from build123d import *

# Parameters (mm, degrees)
BOSS_EXTRUDE1_DEPTH = 25.4
SKETCH2_R           = 2.4892
CUT_EXTRUDE1_DEPTH  = 4.175
SKETCH4_R           = 2.4892
CUT_EXTRUDE2_DEPTH  = 16.875


with BuildPart() as part:
    # Sketch1 → Boss-Extrude1 (new body)
    with BuildSketch(Plane.XY):
        Polygon((0, 0), (0, 38.1), (3.175, 38.1), (3.175, 3.175), (15.875, 3.175), (15.875, 0), align=None)
    extrude(amount=BOSS_EXTRUDE1_DEPTH)

    # Sketch2 → Cut-Extrude1 (cut, through all)
    with BuildSketch(Plane(origin=(0, 3.175, 0), x_dir=(1, 0, 0), z_dir=(0, 1, 0))):
        with Locations((9.525, -6.35)):
            Circle(SKETCH2_R)
        with Locations((9.525, -19.05)):
            Circle(SKETCH2_R)
    extrude(amount=-CUT_EXTRUDE1_DEPTH, mode=Mode.SUBTRACT)

    # Sketch4 → Cut-Extrude2 (cut, through all)
    with BuildSketch(Plane.ZY):
        with Locations((6.35, 31.75)):
            Circle(SKETCH4_R)
        with Locations((19.05, 31.75)):
            Circle(SKETCH4_R)
        with Locations((19.05, 19.05)):
            Circle(SKETCH4_R)
        with Locations((6.35, 19.05)):
            Circle(SKETCH4_R)
    extrude(amount=-CUT_EXTRUDE2_DEPTH, mode=Mode.SUBTRACT)


solid = part.part
Design review of the part built by this model. Coordinates are the model's own, in mm. A direction names the side the tool comes from. Round coordinates to 2 decimals unless told otherwise and drop trailing zeros. Write each loop counter-clockwise with the first axis right and the second up, starting at its lowest first coordinate (ties: lowest second). Pieces come first, ordered by that corner, then holes.
Item 1: Wall thickness on L1, parallel to Y at x = 1.9, z = 19.05; L2, parallel to X at y = 1.05, z = 19.05 (3 decimals); L3, parallel to Y at x = 5, z = 7.25 (3 decimals): over which ranges is each line inside the solid? List them lowest first.
Item 2: For faces 1 (the flat face through (9, 3.175, 13)), 2 (the flat face through (0, 19, 13)), list the 3-axis set-ups (+Z, -Z, +X, -X, +Y, -Y) from which the entire face can be reached by the end or side of a thin tool; tool diameter is ignored.
Item 3: Consider section D-D on z = 12.5. Give the boundary of the cut face in (x, y) (3 decimals).
Item 4: Consider section A-A on z = 19.05. Give the boundary of the cut face in (x, y) (3 decimals).
Item 5: Consider section C-C on y = 19.05. Give the boundary of the cut face in (x, z) (3 decimals).
Item 6: Draft analysis for pull direction Y (two halves, no side actions). For faces 3 (the cylindrical face through (1.565, 31.859, 16.563)), 4 (the flat face through (3.175, 21, 13)), 5 (the flat face through (2, 38.1, 13)), state which applies: released by +Y, released by -Y, zero draft, split by the parting line, or undercut.
Item 7: For pin 1 Ø3 at (x, z) = (9.525, 6.35) entering from +Y; pin 2 Ø4 at (x, z) = (7, 8) entering from +Y (3 decimals); pin 3 Ø5 at (y, z) = (23.5, 18) entering from +X (3 decimals), all flat-tipped, find the tip position at first contact; note any pin that passes through.
Item 8: Consider section B-B on x = 10.25. Give the boundary of the cut face in (y, z) (3 decimals), and give its area (3 significant figures).
Check values:
1. L1: y = 0 to 16.56, 21.54 to 29.26, 34.24 to 38.1
1. L2: x = 0 to 7.036, 12.014 to 15.875
1. L3: y = 0 to 3.175
2. face 1: +Z, -Z, +X, +Y
2. face 2: +Z, -Z, -X, +Y, -Y
3. outline: (0, 0) - (15.875, 0) - (15.875, 3.175) - (3.175, 3.175) - (3.175, 38.1) - (0, 38.1) - close
4. outline: (0, 0) - (7.036, 0) - (7.036, 3.175) - (3.175, 3.175) - (3.175, 16.561) - (0, 16.561) - close; (0, 21.539) - (3.175, 21.539) - (3.175, 29.261) - (0, 29.261) - close; (0, 34.239) - (3.175, 34.239) - (3.175, 38.1) - (0, 38.1) - close; (12.014, 0) - (15.875, 0) - (15.875, 3.175) - (12.014, 3.175) - close
5. outline: (0, 0) - (3.175, 0) - (3.175, 3.861) - (0, 3.861) - close; (0, 8.839) - (3.175, 8.839) - (3.175, 16.561) - (0, 16.561) - close; (0, 21.539) - (3.175, 21.539) - (3.175, 25.4) - (0, 25.4) - close
6. face 3: undercut
6. face 4: zero draft
6. face 5: released by +Y
7. pin 1: passes through
7. pin 2: stops at y = 3.175
7. pin 3: stops at x = 3.175
8. outline: (0, 0) - (3.175, 0) - (3.175, 3.969) - (0, 3.969) - close; (0, 8.731) - (3.175, 8.731) - (3.175, 16.669) - (0, 16.669) - close; (0, 21.431) - (3.175, 21.431) - (3.175, 25.4) - (0, 25.4) - close
8. area: 50.4 mm2
